```python
from build123d import *

# Parameters (mm, degrees)
SKETCH1_W                = 0.566
SKETCH1_H                = 1
M3_CLEARANCE_HOLE1_D     = 3.4
M3_CLEARANCE_HOLE1_DEPTH = 8.566
M3_CLEARANCE_HOLE1_TIP   = 1.021463052
CHAMFER1_SIZE            = 2
BOSS_EXTRUDE1_DEPTH      = 35
SKETCH9_R                = 1.7
CUT_EXTRUDE1_DEPTH       = 10


with BuildPart() as part:
    # Sketch1 → Revolve17 (revolve)
    with BuildSketch(Plane.XY, mode=Mode.PRIVATE) as revolve17_sk:
        Polygon((14.13111535, 39), (14.13111535, 34.5), (22.03011535, 34.5), (22.03011535, 36), (22.69711535, 36), (22.69711535, 39), align=None)
        Polygon((-14.010170791, 3.15), (-14.010170791, 3.8), (-18.343504124, 3.15), (-18.343504124, 1.9), (0, 1.9), (21.56511535, 21.5), (22.13111535, 21.5), (22.13111535, 22.5), (22.13111535, 24.5), (22.69711535, 24.5), (22.69711535, 34), (22.03011535, 34), (22.03011535, 34.5), (14.13111535, 34.5), (14.13111535, 21.5), (-5.343504124, 3.8), (-9.676837458, 3.15), (-9.676837458, 3.8), align=None)
        with Locations((22.41411535, 22)):
            Rectangle(SKETCH1_W, SKETCH1_H)
    revolve(revolve17_sk.sketch.rotate(Axis((-801.927103621, 0, 0), (1, 0, 0)), 90), axis=Axis((-801.927103621, 0, 0), (1, 0, 0)))

    # M3 Clearance Hole1
    with Locations(Plane.ZY.offset(-14.13111535)):
        with Locations((0, -30.5), (0, 30.5), (30.5, 0), (-30.5, 0)):
            Hole(M3_CLEARANCE_HOLE1_D / 2, depth=M3_CLEARANCE_HOLE1_DEPTH)
            with Locations((0, 0, -(M3_CLEARANCE_HOLE1_DEPTH + M3_CLEARANCE_HOLE1_TIP / 2))):  # 118° drill point
                Cone(0, M3_CLEARANCE_HOLE1_D / 2, M3_CLEARANCE_HOLE1_TIP, mode=Mode.SUBTRACT)

    # Chamfer1
    chamfer1_edges = [part.edges().sort_by_distance(p)[0] for p in [
        (14.13111535, 0, -39),
    ]]
    chamfer(chamfer1_edges, length=CHAMFER1_SIZE)

    # Sketch1<11> → Boss-Extrude1 (add, symmetric)
    with BuildSketch(Plane.XY):
        Polygon((14.13111535, 39), (14.13111535, 34.5), (22.03011535, 34.5), (22.03011535, 36), (22.69711535, 36), (22.69711535, 39), align=None)
    extrude(amount=BOSS_EXTRUDE1_DEPTH, both=True)

    # Sketch9 → Cut-Extrude1 (cut)
    with BuildSketch(Plane(origin=(0, 34.5, 0), x_dir=(-1, 0, 0), z_dir=(0, -1, 0))):
        with Locations(Location((-18.08061535, -31, 0), (0, 0, 90))):
            Circle(SKETCH9_R)
        with Locations((-18.08061535, 31)):
            Circle(SKETCH9_R)
    extrude(amount=-CUT_EXTRUDE1_DEPTH, mode=Mode.SUBTRACT)


solid = part.part
```
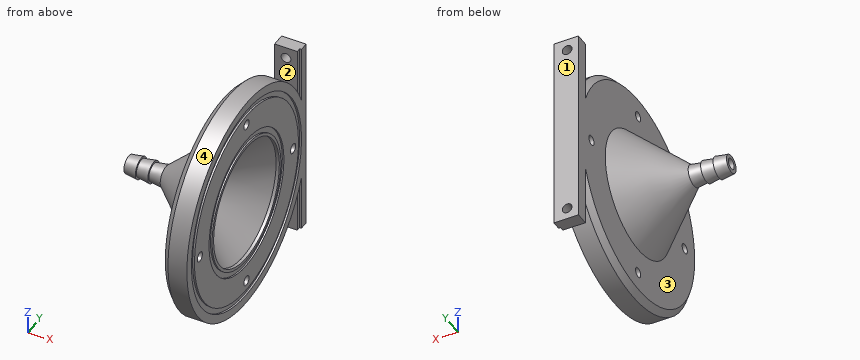
Model file for the job. Use its own axes, mm. Face numbers are marked on the shaded views. Coordinates: 2 decimals unless noted, no trailing zeros. Write each loop counter-clockwise with the first axis right and the second up, starting at its lowest first coordinate (ties: lowest second). Pieces come first, ordered by that corner, then holes. Notation, with made-up numbers: (-11.5, 87.5) - (43.5, 87.5) arc R24 ccw to (43.5, 120.5) - close; hole circle Ø5 at (14.5, 10.5). An arc over 180 degrees is marked (long way). One line per question, with ' | ' between items. Start each with the question number.
Q1. Pull direction Y, two halves, no side cores. Call the marked faces 1, 2, 3 and 4: pulls with the +Y half, pulls with the -Y half, needs draft (parallel to the pull), parting line crosses it, or undercut.
Q2. Drill centre lines: line 1 (Y direction, x = 22, z = 0); line 2 (X direction, y = -3, z = -26.5); line 3 (Y direction, x = 16.5, z = -21). Where is each one in solid material? Low to high. Write a range as [from, to].
Q3. Pin check, flat tips, straight feed: pin 1 (1.2 mm diameter, centred on y = 35, z = -25, fed in from +X); pin 2 (2 mm diameter, centred on x = 11, z = 12.5, fed in from -Y); pin 3 (6 mm diameter, centred on y = 27, z = -22, fed in from -X); pin 4 (2 mm diameter, centred on y = 0, z = 30.5, fed in from +X). Stop position of each tip, or through.
Q4. Cut at A-A, the plane y = 0. Give the number of separate pieces and of enclosed holes in the cut face, then the cut area to 3 significant figures.
Q5. Cut at C-C, the plane x = 10.5. List the corners of the cut face in (y, z), then the cut area to 3 significant figures.
Answer below:
1) face 1: pulls with the +Y half | face 2: undercut | face 3: needs draft | face 4: undercut
2) line 1: [-39, -32.2], [-28.8, -21.5], [21.5, 28.8], [32.2, 39] | line 2: [14.13, 22.7] | line 3: [-32.86, 32.86], [34.5, 39]
3) pin 1: x = 22.03 | pin 2: y = -15.3 | pin 3: x = 14.13 | pin 4: through
4) separate pieces: 4 | enclosed holes: 0 | area: 561 mm^2
5) outline: circle Ø36.4 at (0, 0); hole circle Ø22.89 at (0, 0) | area: 629 mm^2
